Part model, mm, in its own coordinate system. Give positions to 0.01 mm unless a question says otherwise; leave off trailing zeros. Order: outer loops, then holes, each group sorted by start corner. A loop starts at its lowest first (then second) coordinate and runs counter-clockwise, first axis right, second up. Notation, with made-up numbers: M 26,82.5 L 30,82.5 A22 ccw 30,89.5 Z; hole C 38,-37.75 d3. An arc over 180 degrees is marked long. Return JSON: item names as keys, results as strings.
from build123d import *

# Parameters (mm, degrees)
F1_DEPTH = 12.7
F2_R     = 3.175
F3_DEPTH = 25.4
F4_R     = 6.35
F5_DEPTH = 25.4
F6_R     = 3.175
F7_DEPTH = 19.05


with BuildPart() as f1:
    # F0 (on Top) → F1 (new body)
    with BuildSketch(Plane.XY):
        Polygon((64.839908, 16.544953), (0, 16.544953), (-43.110092, 16.544953), (-43.110092, -34.255047), (64.839908, -34.255047), align=None)
    extrude(amount=F1_DEPTH)

    # F2 (on face) → F3 (cut)
    with BuildSketch(Plane.XY.offset(12.7)):
        with Locations((-5.010092, -21.555047)):
            Circle(F2_R)
        with Locations((-5.010092, 3.844953)):
            Circle(F2_R)
        with Locations((52.139908, 3.844953)):
            Circle(F2_R)
        with Locations((52.139908, -21.555047)):
            Circle(F2_R)
    extrude(amount=-F3_DEPTH, mode=Mode.SUBTRACT)

    # F4 (on face) → F5 (cut)
    with BuildSketch(Plane.XY.offset(12.7)):
        with Locations((-30.410092, -2.505047)):
            Circle(F4_R)
    extrude(amount=-F5_DEPTH, mode=Mode.SUBTRACT)

    # F6 (on face) → F7 (cut)
    with BuildSketch(Plane(origin=(0, 16.544953, 0), x_dir=(-1, 0, 0), z_dir=(0, 1, 0))):
        with Locations((30.410092, 6.35)):
            Circle(F6_R)
    extrude(amount=-F7_DEPTH, mode=Mode.SUBTRACT)


solid = f1.part
Q1. Two-plate mould, pull along Z, no slides. Class faces 1 (the cylindrical face through (-7.53, 1.913, 6.439)), 2 (the cylindrical face through (-32.117, 9.864, 9.027)), 3 (the flat face through (10, -8, 12.7)): +Z half, -Z half, draft (parallel to the pull), parting line (faces both ways), or undercut.
Established:
{"face 1": "draft", "face 2": "undercut", "face 3": "+Z half"}
Q2. Band-saw the part on A-A (x = 53). Give the cut face in (y, z).
Established:
{"outline": "M -34.26,0 L -24.61,0 L -24.61,12.7 L -34.26,12.7 Z; M -18.5,0 L 0.79,0 L 0.79,12.7 L -18.5,12.7 Z; M 6.9,0 L 16.54,0 L 16.54,12.7 L 6.9,12.7 Z"}
Q3. Band-saw the part on D-D (z = 6.35). Give the cut face in (x, y) (3 decimals), then the cut area to 3 significant figures.
Established:
{"outline": "M -43.11,-34.255 L 64.84,-34.255 L 64.84,16.545 L -27.235,16.545 L -27.235,2.994 A6.35 cw long -33.585,2.994 L -33.585,16.545 L -43.11,16.545 Z; hole C -5.01,-21.555 d6.35; hole C -5.01,3.845 d6.35; hole C 52.14,-21.555 d6.35; hole C 52.14,3.845 d6.35", "area": "5,150 mm²"}
Q4. Band-saw the part on C-C (z = 11.25). Give the cut face in (x, y) (3 decimals).
Established:
{"outline": "M -43.11,-34.255 L 64.84,-34.255 L 64.84,16.545 L -43.11,16.545 Z; hole C -30.41,-2.505 d12.7; hole C -5.01,-21.555 d6.35; hole C -5.01,3.845 d6.35; hole C 52.14,-21.555 d6.35; hole C 52.14,3.845 d6.35"}
Q5. Probe line 1 along X through (y, z) = (-21.5, 6.75); line 2 along X through (y, z) = (5, 5.5); line 3 along X through (y, z) = (-5, 2.5). List the from-to ranges inside material, lowest first.
Established:
{"line 1": "x = -43.11 to -8.18, -1.84 to 48.97, 55.31 to 64.84", "line 2": "x = -43.11 to -33.47, -27.35 to -7.97, -2.05 to 49.18, 55.1 to 64.84", "line 3": "x = -43.11 to -36.25, -24.57 to 64.84"}
Q6. Band-saw the part on B-B (y = -4). Give the cut face in (x, z).
Established:
{"outline": "M -43.11,0 L -36.58,0 L -36.58,12.7 L -43.11,12.7 Z; M -24.24,0 L 64.84,0 L 64.84,12.7 L -24.24,12.7 Z"}
Q7. Pin check, flat tip, straight feed: pin 1 (5.5 mm diameter, centred on x = -5.01, y = -21.56, fed in from +Z). Stop position of the tip, or through.
Established:
{"pin 1": "passes through"}
